Geometry check sheet. Reference: the model listing, model coordinates, mm. A direction names the side the tool comes from. Coordinates: 2 decimals unless noted, no trailing zeros. Write each loop counter-clockwise with the first axis right and the second up, starting at its lowest first coordinate (ties: lowest second). Pieces come first, ordered by that corner, then holes. Notation, with made-up numbers: M 46.25,-22 L 74.25,-22 A18 ccw 74.25,11 Z; hole C 72.5,4.5 d6. An arc over 180 degrees is marked long. Write each question's results on one line, items separated by ' | '.
```python
from build123d import *

# Parameters (mm, degrees)
F0_R      = 2.5
F1_DEPTH  = 2
F2_R      = 4.5
F3_DEPTH  = 9
F4_R      = 1.718291
F5_DEPTH  = 6
F6_R      = 1
F7_R      = 1.975543
F8_DEPTH  = 3
F9_R      = 1.277831
F10_DEPTH = 2


with BuildPart() as f1:
    # F0 (on Top) → F1 (new body)
    with BuildSketch(Plane.XY):
        Circle(F0_R)
    extrude(amount=F1_DEPTH)

    # F2 (on face) → F3 (join)
    with BuildSketch(Plane.XY.offset(2)):
        Circle(F2_R)
    extrude(amount=F3_DEPTH)

    # F4 (on face) → F5 (cut)
    with BuildSketch(Plane(origin=(0, 0, 0), x_dir=(1, 0, 0), z_dir=(0, 0, -1))):
        Circle(F4_R)
    extrude(amount=-F5_DEPTH, mode=Mode.SUBTRACT)

    # F6
    f6_edges = [f1.edges().sort_by_distance(p)[0] for p in [
        (-4.5, 0, 11),
        (-4.5, 0, 2),
    ]]
    fillet(f6_edges, radius=F6_R)

    # F7 (on face) → F8 (join)
    with BuildSketch(Plane.XY.offset(11)):
        Circle(F7_R)
    extrude(amount=F8_DEPTH)

    # F9 (on face) → F10 (cut)
    with BuildSketch(Plane.XY.offset(14)):
        Circle(F9_R)
    extrude(amount=-F10_DEPTH, mode=Mode.SUBTRACT)


solid = f1.part
```
Q1. Scan lines: probe 1 along Y at (x, z) = (0, 13.45); probe 2 along Z at (x, y) = (3, -0.25); probe 3 along Y at (x, z) = (0.25, 3). Record each from-to range of solid material in increasing order.
Geometry check:
probe 1: y = -1.98 to -1.28, 1.28 to 1.98 | probe 2: z = 2 to 11 | probe 3: y = -4.49 to -1.7, 1.7 to 4.49
Q2. Sectioned sample at A-A on y = 0. Record the cut outline in (x, z), and give its area (3 significant figures).
Geometry check:
outline: M -4.5,3 A1 ccw -3.5,2 L -2.5,2 L -2.5,0 L -1.72,0 L -1.72,6 L 1.72,6 L 1.72,0 L 2.5,0 L 2.5,2 L 3.5,2 A1 ccw 4.5,3 L 4.5,10 A1 ccw 3.5,11 L 1.98,11 L 1.98,14 L 1.28,14 L 1.28,12 L -1.28,12 L -1.28,14 L -1.98,14 L -1.98,11 L -3.5,11 A1 ccw -4.5,10 Z | area: 76.3 mm2
Q3. Depth check by flat-ended pin: P1, Ø3.5, axis at x = -1, y = -1.5, coming from the -Z side; P2, Ø3, axis at x = -3, z = 9, coming from the +Y side; P3, Ø4, axis at x = 2.5, z = 12.5, coming from the +Y side; P4, Ø1, axis at x = 0, y = -0.5, coming from the -Z side. Enter the tip coordinate at first touch or a pass-through.
Geometry check:
P1: stops at z = 0 | P2: stops at y = 4.24 | P3: stops at y = 3.89 | P4: stops at z = 6
Q4. Sectioned sample at C-C on z = 9.5. Record the cut outline in (x, y).
Geometry check:
outline: C 0,0 d9
Q5. Access from +Z, -Z, +X, -X, +Y, -Y to the whole of each face (thin tool, end or side, straight path). Record for faces 1 (the flat face through (2, -2, 11)), 2 (the cylindrical face through (-0.54, -2.44, 0.99)), 3 (the flat face through (-1, -2, 0)).
Geometry check:
face 1: +Z | face 2: -Z | face 3: -Z, +X, -X, +Y, -Y
Q6. Mould release check, pull along X, two halves, no side actions. Record for faces 4 (the cylindrical face through (-0.59, 4.46, 6.45)), 5 (the flat face through (0, 0, 12)), 6 (the flat face through (2, -2, 2)): pulls with the +X half, pulls with the -X half, needs draft (parallel to the pull), parting line crosses it, or undercut.
Geometry check:
face 4: parting line crosses it | face 5: undercut | face 6: needs draft
